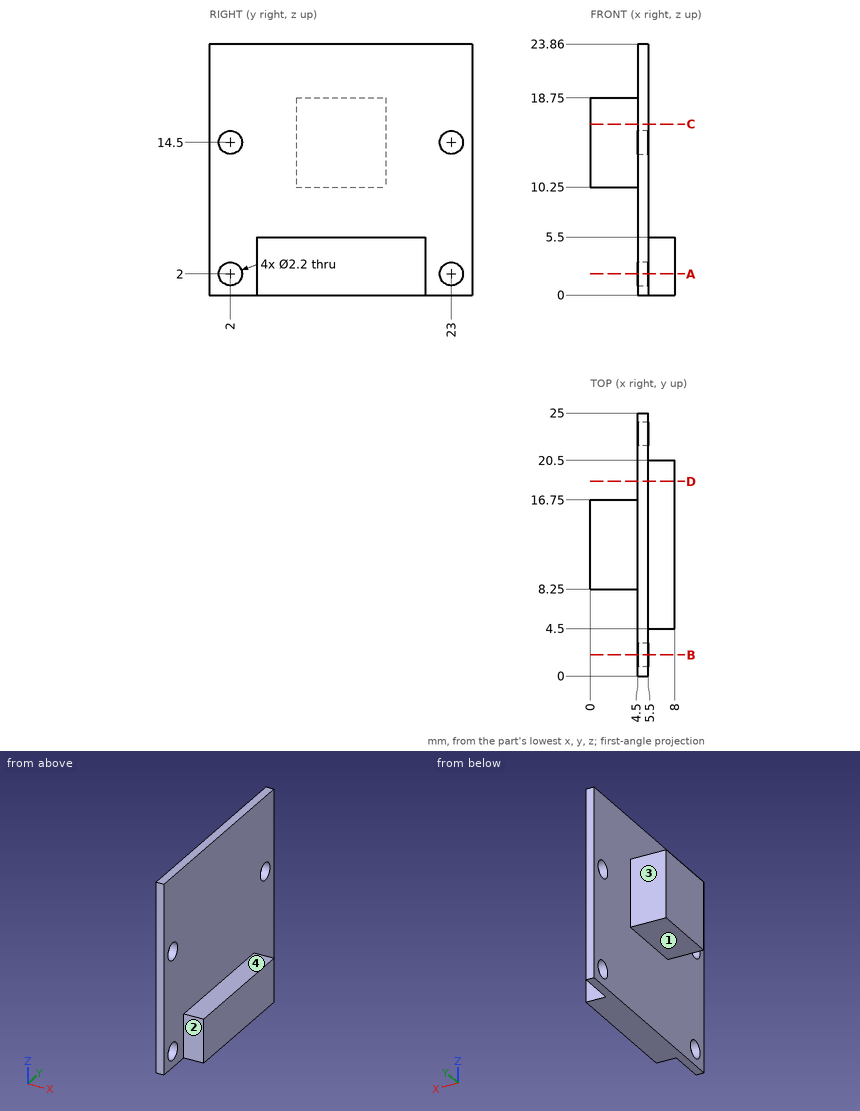
Study the drawing (mm; zero at the part's minimum x, y, z) and answer. A direction names the side the tool comes from. Give positions to 0.01 mm unless a question says otherwise; leave off trailing zeros. Write each loop counter-clockwise with the first axis right and the second up, starting at its lowest first coordinate (ties: lowest second). Pieces come first, ordered by that corner, then holes. Notation, with made-up numbers: (-35, 82) - (-15, 82) arc R21 cw to (-15, 93) - close; hole circle Ø11 at (56, 69). An arc over 180 degrees is marked (long way). Write item = value, one per line. Start each with the question number.
Item 1: A tool of negligible diameter and unlimited length cuts with its end or side. For the marked faces 1, 2, 3 and 4, from which of +Z, -Z, +X, -X, +Y, -Y can it reach the whole face along a straight path? Write none if from no direction.
Item 2: Find the intervals of material crossed by probe 1 along Z at (x, y) = (5, 23); probe 2 along Y at (x, z) = (5, 2); probe 3 along X at (y, z) = (16, 22), in increasing order. Write a range as [from, to].
Item 3: Find section B-B (y = 2). Give the vertices of the cut face in (x, z), then the cut area to 3 significant figures.
Item 4: Each of these flat-tipped pins is pushed along its axis until it touches: P1, Ø1, axis at y = 9.5, z = 16, coming from the +X side; P2, Ø1.8, axis at y = 23, z = 14.5, coming from the +X side; P3, Ø3, axis at y = 22, z = 19.5, coming from the -X side; P4, Ø1.3, axis at x = 2.5, y = 11.5, coming from the -Z side. Where does it stop, or does it pass through?
Item 5: Find section D-D (y = 18.5). Give the vertices of the cut face in (x, z).
Item 6: Find section A-A (z = 2). Give the vertices of the cut face in (x, y), then the cut area to 3 significant figures.
Item 7: Find section C-C (z = 16.25). Give the vertices of the cut face in (x, y), then the cut area to 4 significant figures.
Response:
q1.face_1 = -Z, -X, +Y, -Y
q1.face_2 = +Z, -Z, +X, -Y
q1.face_3 = +Z, -Z, -X, +Y
q1.face_4 = +Z, +X, +Y, -Y
q2.probe_1 = [0, 0.9], [3.1, 13.4], [15.6, 23.86]
q2.probe_2 = [0, 0.9], [3.1, 21.9], [24.1, 25]
q2.probe_3 = [4.5, 5.5]
q3.outline = (4.5, 0) - (5.5, 0) - (5.5, 0.9) - (4.5, 0.9) - close; (4.5, 3.1) - (5.5, 3.1) - (5.5, 13.4) - (4.5, 13.4) - close; (4.5, 15.6) - (5.5, 15.6) - (5.5, 23.86) - (4.5, 23.86) - close
q3.area = 19.5 mm²
q4.P1 = 5.5
q4.P2 = through
q4.P3 = 4.5
q4.P4 = 10.25
q5.outline = (4.5, 0) - (8, 0) - (8, 5.5) - (5.5, 5.5) - (5.5, 23.86) - (4.5, 23.86) - close
q6.outline = (4.5, 0) - (5.5, 0) - (5.5, 0.9) - (4.5, 0.9) - close; (4.5, 3.1) - (5.5, 3.1) - (5.5, 4.5) - (8, 4.5) - (8, 20.5) - (5.5, 20.5) - (5.5, 21.9) - (4.5, 21.9) - close; (4.5, 24.1) - (5.5, 24.1) - (5.5, 25) - (4.5, 25) - close
q6.area = 60.6 mm²
q7.outline = (0, 8.25) - (4.5, 8.25) - (4.5, 0) - (5.5, 0) - (5.5, 25) - (4.5, 25) - (4.5, 16.75) - (0, 16.75) - close
q7.area = 63.25 mm²
